Read the model definition and answer for the solid it produces. Units are mm, in the model's axes. A direction names the side the tool comes from. Coordinates: 2 decimals unless noted, no trailing zeros. Order: outer loops, then holes, each group sorted by start corner. A loop starts at its lowest first (then second) coordinate and runs counter-clockwise, first axis right, second up. Notation, with made-up numbers: (-26.75, -39) - (7.25, -39) arc R20 ccw to (7.25, -30) - close; hole circle Ø4 at (27, 66.25). An arc over 180 degrees is marked (long way). Answer as a JSON object with one key per item and string values. Group by question number.
from build123d import *

# Parameters (mm, degrees)
CONG_1_R = 0.6


with BuildPart() as part:
    # Esquisse1 → Révolution1 (revolve)
    with BuildSketch(Plane.XY, mode=Mode.PRIVATE) as r_volution1_sk:
        Polygon((0, 4), (11.7, 4), (11.7, 13), (7.7, 13), (7.7, 8), (0, 8), align=None)
    revolve(r_volution1_sk.sketch.rotate(Axis((0, 0, 0), (1, 0, 0)), 90), axis=Axis((0, 0, 0), (1, 0, 0)))

    # Congé1
    cong_1_edges = [part.edges().sort_by_distance(p)[0] for p in [
        (7.7, 0, -13),
        (11.7, 0, -13),
    ]]
    fillet(cong_1_edges, radius=CONG_1_R)


solid = part.part
1. A cutting plane is placed at A-A on z = 0. Write down the section's boundary in (x, y), and give its area (3 significant figures).
2. Straight lines are drawn through the part: L1, parallel to Y at x = 4, z = 0; L2, parallel to X at y = 8.5, z = 1.5; L3, parallel to Y at x = 9, z = 0. For each, find the intervals that lie inside material, in ascending order.
3. For a pull along Y with two mould halves and no side action, classify faces 1 (the cylindrical face through (5.932, 3.905, -0.867)), 2 (the flat face through (11.7, -3, 3)), 3 (the cylindrical face through (9.68, 7.91, -10.316)) as pulls with the +Y half, pulls with the -Y half, needs draft (parallel to the pull), parting line crosses it, or undercut.
4. For faces 4 (the flat face through (0, 2, -4)), 5 (the flat face through (7.7, 3, 8)), determine the directions among +Z, -Z, +X, -X, +Y, -Y from which every point of the face is accessible in a straight line to the end or side of a thin tool.
5. Given pin 1 (4 mm diameter, centred on x = 3.5, y = -5, fed in from +Z); pin 2 (5 mm diameter, centred on y = 0, z = 0, fed in from -X); pin 3 (1 mm diameter, centred on x = 2, z = 7.5, fed in from +Y); pin 4 (2 mm diameter, centred on x = 6.5, z = 5.5, fed in from +Y), each flat-ended and moving along its own axis, determine where each tip first touches the part or whether it passes through.
6. A cutting plane is placed at C-C on x = 5.25. Write down the section's boundary in (y, z).
Derived:
{
 "1": {"outline": "(0, -8) - (7.7, -8) - (7.7, -12.4) arc R0.6 ccw to (8.3, -13) - (11.1, -13) arc R0.6 ccw to (11.7, -12.4) - (11.7, -4) - (0, -4) - close; (0, 4) - (11.7, 4) - (11.7, 12.4) arc R0.6 ccw to (11.1, 13) - (8.3, 13) arc R0.6 ccw to (7.7, 12.4) - (7.7, 8) - (0, 8) - close", "area": "133 mm2"},
 "2": {"L1": "y = -8 to -4, 4 to 8", "L2": "x = 7.7 to 11.7", "L3": "y = -13 to -4, 4 to 13"},
 "3": {"face 1": "undercut", "face 2": "needs draft", "face 3": "parting line crosses it"},
 "4": {"face 4": "+Z, -Z, -X, +Y, -Y", "face 5": "-X"},
 "5": {"pin 1": "stops at z = 7.42", "pin 2": "passes through", "pin 3": "stops at y = 3.87", "pin 4": "stops at y = 6.61"},
 "6": {"outline": "circle Ø16 at (0, 0); hole circle Ø8 at (0, 0)"}
}
